Design review of the part built by this model. Coordinates are the model's own, in mm. A direction names the side the tool comes from. Coordinates: 2 decimals unless noted, no trailing zeros. Write each loop counter-clockwise with the first axis right and the second up, starting at its lowest first coordinate (ties: lowest second). Pieces come first, ordered by that corner, then holes. Notation, with made-up numbers: (28.5, -17.5) - (82.5, -17.5) arc R31 ccw to (82.5, 19.5) - close; hole circle Ø6 at (69.25, -17). An arc over 180 degrees is marked (long way). Answer as CSV lines item,"result". Start each with the question number.
Q1. We need section C-C (x = 33.5). Write out the cut boundary in (y, z), plus the area to 3 significant figures.
Q2. We need section B-B (y = -9.5). Write out the cut boundary in (x, z), plus the area to 3 significant figures.
Q3. Clearance check with flat-ended pins moving along their axes: pin 1 (1 mm diameter, centred on y = 49.5, z = 9, fed in from +X); pin 2 (11 mm diameter, centred on x = 0, z = 26.5, fed in from -Y); pin 3 (4 mm diameter, centred on x = -20, y = 43, fed in from +Z). State where each tip first meets the part, or that it passes through.
Q4. We need section A-A (z = 21.75). Write out the cut boundary in (x, y), plus the area to 3 significant figures.
Q5. We need section D-D (z = 15.75). Write out the cut boundary in (x, y), plus the area to 3 significant figures.
Q6. For line 1 along Z through (x, y) = (-16.5, 48.5); line 2 along Y through (x, z) = (1.5, 19.25); line 3 along X through (y, z) = (-43.5, 12.75), list the stretches that pass through material, from the lowest coordinate up. Write a range as [from, to].
Q7. Machinability: for faces 1 (the face through (25.551, 0, 25)), 2 (the face through (0, -33.094, 25)), 3 (the face through (0, 33.094, 25)), which of the approach directions +Z, -Z, +X, -X, +Y, -Y give a long, thin tool a straight path to every point of the face, cutting with its end or side? Answer none if there is none.
from build123d import *

# Parameters (mm, degrees)
F1_DEPTH = 20
F3_DEPTH = 10


with BuildPart() as f1:
    # F0 (on Top) → F1 (new body)
    with BuildSketch(Plane.XY):
        with BuildLine():
            ThreePointArc((-22.126984, -53.408383), (0, -60.085769), (22.126984, -53.408383))
            ThreePointArc((22.126984, -53.408383), (52.490427, -7.67724), (41, 46))
            ThreePointArc((41, 46), (0, 67.381824), (-41, 46))
            ThreePointArc((-41, 46), (-52.490427, -7.67724), (-22.126984, -53.408383))
        make_face()
    extrude(amount=F1_DEPTH)

    # F2 (on face) → F3 (join)
    with BuildSketch(Plane.XY.offset(20)):
        with BuildLine():
            ThreePointArc((25.551237, 13.094417), (19.693373, 27.236553), (5.551237, 33.094417))
            Line((5.551237, 33.094417), (-5.551237, 33.094417))
            ThreePointArc((-5.551237, 33.094417), (-19.693373, 27.236553), (-25.551237, 13.094417))
            Line((-25.551237, 13.094417), (-25.551237, -13.094417))
            ThreePointArc((-25.551237, -13.094417), (-19.693373, -27.236553), (-5.551237, -33.094417))
            Line((-5.551237, -33.094417), (5.551237, -33.094417))
            ThreePointArc((5.551237, -33.094417), (19.693373, -27.236553), (25.551237, -13.094417))
            Line((25.551237, -13.094417), (25.551237, 13.094417))
        make_face()
    extrude(amount=F3_DEPTH)


solid = f1.part
Results list:
1,outline,"(-44.01, 0) - (54.5, 0) - (54.5, 20) - (-44.01, 20) - close"
1,area,"1,970 mm2"
2,outline,"(-52.12, 0) - (52.12, 0) - (52.12, 20) - (25.55, 20) - (25.55, 30) - (-25.55, 30) - (-25.55, 20) - (-52.12, 20) - close"
2,area,"2,600 mm2"
3,pin 1,"stops at x = 38.73"
3,pin 2,"stops at y = -33.09"
3,pin 3,"stops at z = 20"
4,outline,"(-25.55, -13.09) arc R20 ccw to (-5.55, -33.09) - (5.55, -33.09) arc R20 ccw to (25.55, -13.09) - (25.55, 13.09) arc R20 ccw to (5.55, 33.09) - (-5.55, 33.09) arc R20 ccw to (-25.55, 13.09) - close"
4,area,"3,040 mm2"
5,outline,"(-41, 46) arc R70.73 ccw to (-22.13, -53.41) arc R40 ccw to (22.13, -53.41) arc R70.73 ccw to (41, 46) arc R50 ccw to start"
5,area,"10,700 mm2"
6,line 1,"z = [0, 20]"
6,line 2,"y = [-60.06, 67.36]"
6,line 3,"x = [-33.99, 33.99]"
7,face 1,"+Z, +X, +Y, -Y"
7,face 2,"+Z, +X, -X, -Y"
7,face 3,"+Z, +X, -X, +Y"
